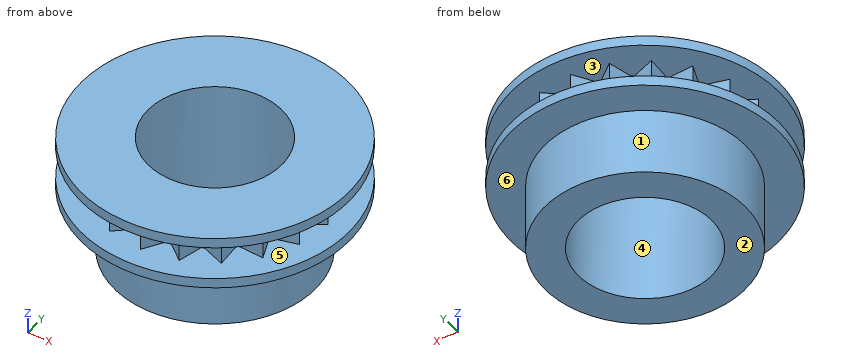
from build123d import *

# Parameters (mm, degrees)
BOSS_EXTRUDE1_DEPTH = 5
SKETCH2_R           = 20
BOSS_EXTRUDE2_DEPTH = 1.5
BOSS_EXTRUDE3_START = 1.5
SKETCH3_R           = 20
BOSS_EXTRUDE3_DEPTH = 1.5
SKETCH4_R           = 13
CUT_EXTRUDE1_DEPTH  = 11.5
SKETCH5_R           = 15
BOSS_EXTRUDE4_DEPTH = 10
CUT_EXTRUDE2_START  = -30
SKETCH6_R           = 13
CUT_EXTRUDE2_DEPTH  = 30
BOSS_EXTRUDE5_START = -18
SKETCH7_R           = 13
SKETCH7_R_2         = 10
BOSS_EXTRUDE5_DEPTH = 18


with BuildPart() as part:
    # Sketch1 → Boss-Extrude1 (new body)
    with BuildSketch(Plane.XY):
        with BuildLine():
            Line((0, 17), (-1.990617103, 13.857757522))
            ThreePointArc((-1.990617103, 13.857757522), (-2.190082511, 13.827636768), (-2.389093211, 13.794645107))
            Line((-2.389093211, 13.794645107), (-5.253288904, 16.167960777))
            Line((-5.253288904, 16.167960777), (-6.175471945, 12.564376079))
            ThreePointArc((-6.175471945, 12.564376079), (-6.355866996, 12.474091339), (-6.534942436, 12.381216715))
            Line((-6.534942436, 12.381216715), (-9.992349289, 13.753288904))
            Line((-9.992349289, 13.753288904), (-9.755828567, 10.041105964))
            ThreePointArc((-9.755828567, 10.041105964), (-9.899494937, 9.899494937), (-10.041105964, 9.755828567))
            Line((-10.041105964, 9.755828567), (-13.753288904, 9.992349289))
            Line((-13.753288904, 9.992349289), (-12.381216715, 6.534942436))
            ThreePointArc((-12.381216715, 6.534942436), (-12.474091339, 6.355866996), (-12.564376079, 6.175471945))
            Line((-12.564376079, 6.175471945), (-16.167960777, 5.253288904))
            Line((-16.167960777, 5.253288904), (-13.794645107, 2.389093211))
            ThreePointArc((-13.794645107, 2.389093211), (-13.827636768, 2.190082511), (-13.857757522, 1.990617103))
            Line((-13.857757522, 1.990617103), (-17, 0))
            Line((-17, 0), (-13.857757522, -1.990617103))
            ThreePointArc((-13.857757522, -1.990617103), (-13.827636768, -2.190082511), (-13.794645107, -2.389093211))
            Line((-13.794645107, -2.389093211), (-16.167960777, -5.253288904))
            Line((-16.167960777, -5.253288904), (-12.564376079, -6.175471945))
            ThreePointArc((-12.564376079, -6.175471945), (-12.474091339, -6.355866996), (-12.381216715, -6.534942436))
            Line((-12.381216715, -6.534942436), (-13.753288904, -9.992349289))
            Line((-13.753288904, -9.992349289), (-10.041105964, -9.755828567))
            ThreePointArc((-10.041105964, -9.755828567), (-9.899494937, -9.899494937), (-9.755828567, -10.041105964))
            Line((-9.755828567, -10.041105964), (-9.992349289, -13.753288904))
            Line((-9.992349289, -13.753288904), (-6.534942436, -12.381216715))
            ThreePointArc((-6.534942436, -12.381216715), (-6.355866996, -12.474091339), (-6.175471945, -12.564376079))
            Line((-6.175471945, -12.564376079), (-5.253288904, -16.167960777))
            Line((-5.253288904, -16.167960777), (-2.389093211, -13.794645107))
            ThreePointArc((-2.389093211, -13.794645107), (-2.190082511, -13.827636768), (-1.990617103, -13.857757522))
            Line((-1.990617103, -13.857757522), (0, -17))
            Line((0, -17), (1.990617103, -13.857757522))
            ThreePointArc((1.990617103, -13.857757522), (2.190082511, -13.827636768), (2.389093211, -13.794645107))
            Line((2.389093211, -13.794645107), (5.253288904, -16.167960777))
            Line((5.253288904, -16.167960777), (6.175471945, -12.564376079))
            ThreePointArc((6.175471945, -12.564376079), (6.355866996, -12.474091339), (6.534942436, -12.381216715))
            Line((6.534942436, -12.381216715), (9.992349289, -13.753288904))
            Line((9.992349289, -13.753288904), (9.755828567, -10.041105964))
            ThreePointArc((9.755828567, -10.041105964), (9.899494937, -9.899494937), (10.041105964, -9.755828567))
            Line((10.041105964, -9.755828567), (13.753288904, -9.992349289))
            Line((13.753288904, -9.992349289), (12.381216715, -6.534942436))
            ThreePointArc((12.381216715, -6.534942436), (12.474091339, -6.355866996), (12.564376079, -6.175471945))
            Line((12.564376079, -6.175471945), (16.167960777, -5.253288904))
            Line((16.167960777, -5.253288904), (13.794645107, -2.389093211))
            ThreePointArc((13.794645107, -2.389093211), (13.827636768, -2.190082511), (13.857757522, -1.990617103))
            Line((13.857757522, -1.990617103), (17, 0))
            Line((17, 0), (13.857757522, 1.990617103))
            ThreePointArc((13.857757522, 1.990617103), (13.827636768, 2.190082511), (13.794645107, 2.389093211))
            Line((13.794645107, 2.389093211), (16.167960777, 5.253288904))
            Line((16.167960777, 5.253288904), (12.564376079, 6.175471945))
            ThreePointArc((12.564376079, 6.175471945), (12.474091339, 6.355866996), (12.381216715, 6.534942436))
            Line((12.381216715, 6.534942436), (13.753288904, 9.992349289))
            Line((13.753288904, 9.992349289), (10.041105964, 9.755828567))
            ThreePointArc((10.041105964, 9.755828567), (9.899494937, 9.899494937), (9.755828567, 10.041105964))
            Line((9.755828567, 10.041105964), (9.992349289, 13.753288904))
            Line((9.992349289, 13.753288904), (6.534942436, 12.381216715))
            ThreePointArc((6.534942436, 12.381216715), (6.355866996, 12.474091339), (6.175471945, 12.564376079))
            Line((6.175471945, 12.564376079), (5.253288904, 16.167960777))
            Line((5.253288904, 16.167960777), (2.389093211, 13.794645107))
            ThreePointArc((2.389093211, 13.794645107), (2.190082511, 13.827636768), (1.990617103, 13.857757522))
            Line((1.990617103, 13.857757522), (0, 17))
        make_face()
    extrude(amount=BOSS_EXTRUDE1_DEPTH)

    # Sketch2 → Boss-Extrude2 (add)
    with BuildSketch(Plane(origin=(0, 0, 0), x_dir=(-1, 0, 0), z_dir=(0, 0, -1))):
        Circle(SKETCH2_R)
    extrude(amount=BOSS_EXTRUDE2_DEPTH)

    # Sketch3 → Boss-Extrude3 (add)
    with BuildSketch(Plane.XY.offset(5).offset(BOSS_EXTRUDE3_START)):
        with Locations(Location((0, 0, 0), (0, 0, 180))):
            Circle(SKETCH3_R)
    extrude(amount=-BOSS_EXTRUDE3_DEPTH)

    # Sketch4 → Cut-Extrude1 (cut)
    with BuildSketch(Plane.XY.offset(6.5)):
        Circle(SKETCH4_R)
    extrude(amount=-CUT_EXTRUDE1_DEPTH, mode=Mode.SUBTRACT)

    # Sketch5 → Boss-Extrude4 (add)
    with BuildSketch(Plane(origin=(0, 0, -1.5), x_dir=(-1, 0, 0), z_dir=(0, 0, -1))):
        Circle(SKETCH5_R)
    extrude(amount=BOSS_EXTRUDE4_DEPTH)

    # Sketch6 → Cut-Extrude2 (cut)
    with BuildSketch(Plane(origin=(0, 0, -11.5), x_dir=(-1, 0, 0), z_dir=(0, 0, -1)).offset(CUT_EXTRUDE2_START)):
        with Locations(Location((0, 0, 0), (0, 0, 180))):
            Circle(SKETCH6_R)
    extrude(amount=CUT_EXTRUDE2_DEPTH, mode=Mode.SUBTRACT)

    # Sketch7 → Boss-Extrude5 (add)
    with BuildSketch(Plane(origin=(0, 0, -11.5), x_dir=(-1, 0, 0), z_dir=(0, 0, -1)).offset(BOSS_EXTRUDE5_START)):
        Circle(SKETCH7_R)
        Circle(SKETCH7_R_2, mode=Mode.SUBTRACT)
    extrude(amount=BOSS_EXTRUDE5_DEPTH)


solid = part.part
Source: CAD feature listing. Evaluate the final solid. Frame: model axes, mm. Face numbers are marked on the shaded views. A direction names the side the tool comes from. Give positions to 0.01 mm unless a question says otherwise; leave off trailing zeros. Loops run counter-clockwise (first coordinate to the right, second up) from the corner with the lowest first, then second, coordinate; pieces in that order, holes last. Notation, with made-up numbers: (88, 29.5) -> (126, 29.5) arc R23 cw to (126, 47.5) -> close; hole circle Ø7 at (85.5, -31). An arc over 180 degrees is marked (long way). Use a Markdown table: item, result. Add a question column.
1) Pull-direction query (Z, two-part tool) for the marked faces 1, 2 and 3; classes: +Z half, -Z half, draft (parallel to the pull), parting line (faces both ways), or undercut.
2) First-contact query: pin 1 (1 mm diameter, centred on x = 13, z = -0.5, fed in from +Y); pin 2 (4 mm diameter, centred on y = -11, z = -5.5, fed in from +X); pin 3 (3 mm diameter, centred on y = 1, z = -6.5, fed in from -X). Flat tips, straight axial feed; report the tip coordinate or a pass-through.
3) Reachability of the marked faces 4, 5 and 6 from +Z, -Z, +X, -X, +Y, -Y: full face, straight path, thin tool, end or side. Return the list, or none.
4) Section query B-B, the plane x = 11.5. Return the cut outline in (y, z), then the cut area to 3 significant figures.
5) Line query: line 1 along Z through (x, y) = (6.5, -18); line 2 along Y through (x, z) = (0, -7.5); line 3 along Y through (x, z) = (0, -1.25). Output: solid intervals per line, ascending. Write a range as [from, to].
6) Section query C-C, the plane z = -3. Return the cut outline in (x, y).
7) Section query A-A, the plane y = -15.5. Return the cut outline in (x, z).
Numbers:
| question | item | result |
|---|---|---|
| 1 | face 1 | draft |
| 1 | face 2 | -Z half |
| 1 | face 3 | undercut |
| 2 | pin 1 | stops at y = 15.61 |
| 2 | pin 2 | stops at x = 12 |
| 2 | pin 3 | stops at x = -15 |
| 3 | face 4 | +Z, -Z |
| 3 | face 5 | none |
| 3 | face 6 | -Z |
| 4 | outline | (-16.36, -1.5) -> (-9.63, -1.5) -> (-9.63, -11.5) -> (9.63, -11.5) -> (9.63, -1.5) -> (16.36, -1.5) -> (16.36, 0) -> (9.85, 0) -> (9.85, 5) -> (16.36, 5) -> (16.36, 6.5) -> (-16.36, 6.5) -> (-16.36, 5) -> (-9.85, 5) -> (-9.85, 0) -> (-16.36, 0) -> close |
| 4 | area | 389 mm2 |
| 5 | line 1 | z = [-1.5, 0], [5, 6.5] |
| 5 | line 2 | y = [-15, -10], [10, 15] |
| 5 | line 3 | y = [-20, -10], [10, 20] |
| 6 | outline | circle Ø30 at (0, 0); hole circle Ø20 at (0, 0) |
| 7 | outline | (-12.64, -1.5) -> (12.64, -1.5) -> (12.64, 0) -> (5.42, 0) -> (5.42, 5) -> (12.64, 5) -> (12.64, 6.5) -> (-12.64, 6.5) -> (-12.64, 5) -> (-5.42, 5) -> (-5.42, 0) -> (-12.64, 0) -> close; hole (-4.45, 0) -> (-0.95, 0) -> (-0.95, 5) -> (-4.45, 5) -> close; hole (0.95, 0) -> (4.45, 0) -> (4.45, 5) -> (0.95, 5) -> close |
